from build123d import *

# Parameters (mm, degrees)
SKETCH_W        = 10
SKETCH_H        = 30
PAD_DEPTH       = 5
THICKNESS_T     = -1
POCKET_DEPTH    = 2
SKETCH002_W     = 10
SKETCH002_H     = 9
POCKET001_DEPTH = 2
PAD001_DEPTH    = 1


with BuildPart() as part:
    # Sketch → Pad (new body)
    with BuildSketch(Plane.XY):
        with Locations((5, 15)):
            Rectangle(SKETCH_W, SKETCH_H)
    extrude(amount=PAD_DEPTH)

    # Thickness
    thickness_openings = [part.faces().sort_by_distance(p)[0] for p in [
        (5, 0, 2.5),
    ]]
    offset(amount=THICKNESS_T, openings=thickness_openings)

    # Sketch001 (on Face5 of Thickness) → Pocket (cut)
    with BuildSketch(Plane.XY.offset(5)):
        with BuildLine():
            Line((3.25, 5.485527), (3.25, 8))
            Line((3.25, 8), (6.75, 8))
            Line((6.75, 8), (6.75, 5.485527))
            ThreePointArc((9.295938, 0), (9.0818, 3.234187), (6.75, 5.485527))
            Line((0.704062, 0), (9.295938, 0))
            ThreePointArc((3.25, 5.485527), (0.9182, 3.234187), (0.704062, 0))
        make_face()
    extrude(amount=-POCKET_DEPTH, mode=Mode.SUBTRACT)

    # Sketch002 (on Face4 of Pocket) → Pocket001 (cut)
    with BuildSketch(Plane(origin=(0, 0, 0), x_dir=(1, 0, 0), z_dir=(0, 0, -1))):
        with Locations((5, -4.5)):
            Rectangle(SKETCH002_W, SKETCH002_H)
    extrude(amount=-POCKET001_DEPTH, mode=Mode.SUBTRACT)

    # Sketch003 (on Face6 of Pocket001) → Pad001 (join)
    with BuildSketch(Plane.XY.offset(5)):
        with BuildLine():
            Line((0, 30), (10, 30))
            Line((10, 30), (10, 5.089746))
            ThreePointArc((10, 5.089746), (8.557562, 6.478447), (6.75, 7.339746))
            Line((6.75, 8), (6.75, 7.339746))
            Line((3.25, 8), (6.75, 8))
            Line((3.25, 7.339746), (3.25, 8))
            ThreePointArc((3.25, 7.339746), (1.442438, 6.478447), (0, 5.089746))
            Line((0, 30), (0, 5.089746))
        make_face()
    extrude(amount=PAD001_DEPTH)


solid = part.part
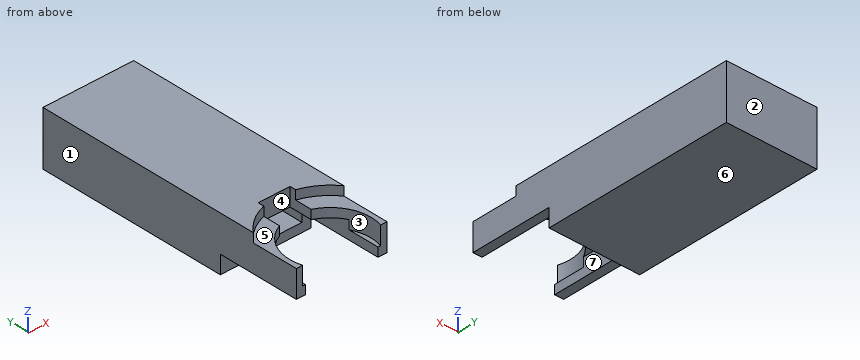
Part model, mm, in its own coordinate system. Face numbers are marked on the shaded views. A direction names the side the tool comes from. Round coordinates to 2 decimals unless told otherwise and drop trailing zeros. Write each loop counter-clockwise with the first axis right and the second up, starting at its lowest first coordinate (ties: lowest second). Pieces come first, ordered by that corner, then holes. Notation, with made-up numbers: M 72,28 L 103,28 A22 cw 103,43 Z; hole C 16.5,-27 d9. An arc over 180 degrees is marked long. Return JSON: item names as keys, results as strings. Group by question number.
(1) Two-plate mould, pull along Y, no slides. Class the marked faces 1, 2, 3 and 4: +Y half, -Y half, draft (parallel to the pull), parting line (faces both ways), or undercut.
(2) Saw through at C-C on z = 3.5. Write the cut outline in (x, y), then the cut area to 3 significant figures.
(3) Saw through at D-D on x = 2.25. Write the cut outline in (y, z), then the cut area to 3 significant figures.
(4) Saw through at B-B on y = 16.75. Write the cut outline in (x, z), then the cut area to 3 significant figures.
(5) Drill centre lines: probe 1 along X at (y, z) = (13.25, 2.55); probe 2 along Z at (x, y) = (2.5, 14.5); probe 3 along Y at (x, z) = (5, 5.05). Where is each one in solid material? Low to high.
(6) Pin check, flat tips, straight feed: pin 1 Ø0.5 at (x, y) = (1, 1.5) entering from +Z; pin 2 Ø1.6 at (x, z) = (4.5, 4.5) entering from -Y; pin 3 Ø0.6 at (x, z) = (7, 1) entering from -Y. Stop position of each tip, or through.
(7) Which spindle directions (+Z, -Z, +X, -X, +Y, -Y) get a long thin tool onto all of the face, cutting with end or side? Do the marked faces 5, 6 and 7. Say none if no direction does.
(8) Saw through at A-A on x = 5.75. Write the cut outline in (y, z).
Returned:
{
 "1": {"face 1": "draft", "face 2": "+Y half", "face 3": "undercut", "face 4": "-Y half"},
 "2": {"outline": "M 0,0 L 0.7,0 A4.5 cw 1,3.4 L 1,29 L 9,29 L 9,3.4 A4.5 cw 9.3,0 L 10,0 L 10,30 L 0,30 Z", "area": "65.5 mm²"},
 "3": {"outline": "M 4.9,4 L 29,4 L 29,1 L 9,1 L 9,0 L 30,0 L 30,6 L 6.95,6 L 6.95,5 L 4.9,5 Z", "area": "72.1 mm²"},
 "4": {"outline": "M 0,0 L 10,0 L 10,6 L 0,6 Z; hole M 1,1 L 9,1 L 9,4 L 1,4 Z", "area": "36.0 mm²"},
 "5": {"probe 1": "0 to 1, 9 to 10", "probe 2": "0 to 1, 4 to 6", "probe 3": "8 to 30"},
 "6": {"pin 1": "z = 3", "pin 2": "y = 8", "pin 3": "y = 9"},
 "7": {"face 5": "+Z, -Y", "face 6": "-Z, +X, -X, +Y, -Y", "face 7": "-Y"},
 "8": {"outline": "M 8,4 L 29,4 L 29,1 L 9,1 L 9,0 L 30,0 L 30,6 L 8,6 Z"}
}
